```python
from build123d import *

# Parameters (mm, degrees)
F0_W     = 300
F0_H     = 300
F1_DEPTH = 20
F2_R     = 11.75
F3_DEPTH = 10
F4_DEPTH = 8.8
F6_DEPTH = 1.2
F7_DEPTH = 4.2


with BuildPart() as f1:
    # F0 (on Top) → F1 (new body)
    with BuildSketch(Plane.XY):
        Rectangle(F0_W, F0_H)
    extrude(amount=F1_DEPTH)

    # F2 (on face) → F3 (cut)
    with BuildSketch(Plane.XY.offset(20)):
        with BuildLine():
            Line((-5, -21.4242852856), (-5, -150))
            Line((-5, -150), (5, -150))
            Line((5, -150), (5, -21.4242852856))
            ThreePointArc((5, -21.4242852856), (0, 22), (-5, -21.4242852856))
        make_face()
        Circle(F2_R, mode=Mode.SUBTRACT)
    extrude(amount=-F3_DEPTH, mode=Mode.SUBTRACT)

    # F2 (on face) → F4 (cut)
    with BuildSketch(Plane.XY.offset(20)):
        with BuildLine():
            Line((-5, -21.4242852856), (-5, -150))
            Line((-5, -150), (5, -150))
            Line((5, -150), (5, -21.4242852856))
            ThreePointArc((5, -21.4242852856), (0, 22), (-5, -21.4242852856))
        make_face()
        Circle(F2_R, mode=Mode.SUBTRACT)
    extrude(amount=-F4_DEPTH, mode=Mode.SUBTRACT)

    # F5 (on face) → F6 (join)
    with BuildSketch(Plane.XY.offset(10)):
        with BuildLine():
            ThreePointArc((5, -21.4242852856), (0, -22), (-5, -21.4242852856))
            Line((-5, -21.4242852856), (-5, -150))
            Line((-5, -150), (5, -150))
            Line((5, -150), (5, -21.4242852856))
        make_face()
    extrude(amount=F6_DEPTH)

    # F2 (on face) → F7 (cut)
    with BuildSketch(Plane.XY.offset(20)):
        Circle(F2_R)
    extrude(amount=-F7_DEPTH, mode=Mode.SUBTRACT)


solid = f1.part
```
Design review of the part built by this model. Coordinates are the model's own, in mm. A direction names the side the tool comes from. Give positions to 0.01 mm unless a question says otherwise; leave off trailing zeros. Order: outer loops, then holes, each group sorted by start corner. A loop starts at its lowest first (then second) coordinate and runs counter-clockwise, first axis right, second up. Notation, with made-up numbers: M 81,52.5 L 139,52.5 A34 ccw 139,90.5 Z; hole C -29.5,68.25 d4. An arc over 180 degrees is marked long. One line per question, with ' | ' between items. Start each with the question number.
Q1. For L1, parallel to Y at x = 0, z = 12; L2, parallel to X at y = 0, z = 17; L3, parallel to Y at x = 0, z = 17.5, list the stretches that pass through material, from the lowest coordinate up. Write a range as [from, to].
Q2. We need section B-B (x = 0). Write out the cut boundary in (y, z), plus the area to 3 significant figures.
Q3. Machinability: for faces 1 (the face through (5, -87, 16)), 2 (the face through (-2, 150, 10)), 3 (the face through (0, 0, 15.8)), which of the approach directions +Z, -Z, +X, -X, +Y, -Y give a long, thin tool a straight path to every point of the face, cutting with its end or side? Answer none if there is none.
Q4. The part is to be moulded in two halves that separate along Y. For faces 4 (the face through (11.207, 3.529, 12.941)), 5 (the face through (-2, 35, 20)), 6 (the face through (9, -9, 10)), 7 (the face through (-2, -150, 10)), say which applies: +Y half, -Y half, draft (parallel to the pull), parting line (faces both ways), or undercut.
Q5. We need section A-A (y = 0). Write out the cut boundary in (x, z), plus the area to 3 significant figures.
Q6. For pin 1 Ø19 at (x, y) = (5.5, 3.5) entering from +Z, flat-tipped, find the tip position at first contact; note if it passes through.
Returned:
1) L1: [-11.75, 11.75], [22, 150] | L2: [-150, -22], [22, 150] | L3: [22, 150]
2) outline: M -150,0 L 150,0 L 150,20 L 22,20 L 22,10 L 11.75,10 L 11.75,15.8 L -11.75,15.8 L -11.75,10 L -22,10 L -22,11.2 L -150,11.2 Z | area: 4,570 mm2
3) face 1: +Z, -Y | face 2: +Z, -Z, +X, -X, +Y | face 3: +Z
4) face 4: undercut | face 5: draft | face 6: undercut | face 7: -Y half
5) outline: M -150,0 L 150,0 L 150,20 L 22,20 L 22,10 L 11.75,10 L 11.75,15.8 L -11.75,15.8 L -11.75,10 L -22,10 L -22,20 L -150,20 Z | area: 5,700 mm2
6) pin 1: z = 15.8
